Work out the finished part from the listing and answer in its coordinate system (mm). Round coordinates to 2 decimals unless told otherwise and drop trailing zeros. Order: outer loops, then holes, each group sorted by start corner. A loop starts at its lowest first (then second) coordinate and runs counter-clockwise, first axis right, second up. Notation, with made-up numbers: M -39.5,68 L -12.5,68 A10 cw -12.5,72 Z; hole C -31,11 d2. An arc over 180 degrees is marked long. Return JSON: item names as keys, results as strings.
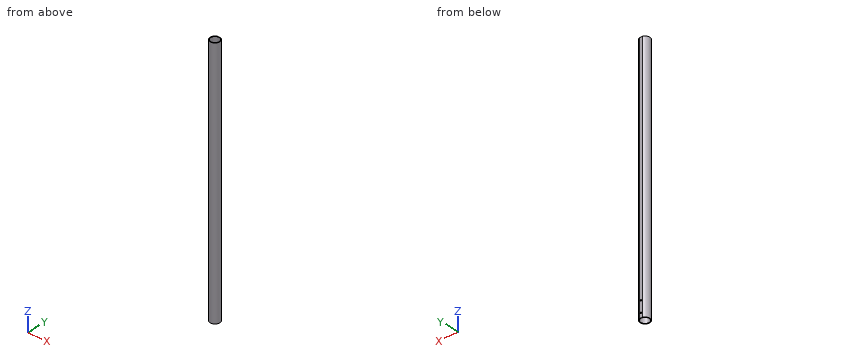
Autodesk Inventor part; units mm, degrees
ref_plane "YZ Plane" through (0, 0, 0) normal (1, 0, 0) x (0, 1, 0)
ref_plane "XZ Plane" through (0, 0, 0) normal (0, 1, 0) x (-1, 0, 0)
ref_plane "XY Plane" through (0, 0, 0) normal (0, 0, 1) x (1, 0, 0)
sketch "Sketch1" plane through (0, 0, 0) normal (0, 0, 1) x (1, 0, 0)
  circle A0 centre (0, 0) radius 11
  circle A1 centre (0, 0) radius 9.38
  dimension "d0" = 22
  dimension "d2" = 1.62
extrude "Extrusion1" add sketch "Sketch1" along normal blind 560
sketch "Sketch6" plane through (0, 0, 560) normal (0, 0, 1) x (1, 0, 0)
  circle A0 centre (0, 0) radius 9.38
  circle A1 centre (0, 0) radius 11
  line L0 (-3.2787, 10.5) -> (3.2787, 10.5)
  dimension "d18" = 10.5
extrude "Extrusion3" cut sketch "Sketch6" against normal through all contours L0 A1 picked at (-0.3693, 10.648)
sketch "Sketch8" plane through (-3.2787, 10.5, 560) normal (0, 1, 0) x (1, 0, 0)
  circle A0 centre (3.2787, 550) radius 1.7934
  point P0 (3.2787, 560)
  dimension "d47" = 10
hole "Hole4" at (0, 10.5, 10) direction (0, -1, 0) diameter 3 depth 8 tip angle 118
sketch "Sketch9" plane through (-3.2787, 10.5, 560) normal (0, 1, 0) x (1, 0, 0)
  circle A0 centre (3.2787, 550) radius 1.5
  circle A1 centre (3.2787, 525) radius 1.2403
  point P0 (3.2787, 560)
  dimension "d55" = 25
hole "Hole5" at (0, 10.5, 35) direction (0, -1, 0) diameter 3 depth 8 tip angle 118
properties part number "2f2barm" material "PVC-Piping"
Item 1: Each of these flat-tipped pins is pushed along its axis until it touches: pin 1 (2.5 mm diameter, centred on x = 0, z = 35, fed in from +Y); pin 2 (4 mm diameter, centred on y = -7, z = 440, fed in from +X); pin 3 (5 mm diameter, centred on y = 4, z = 300.5, fed in from -X). Where does it stop, or does it pass through?
Output:
{"pin 1": "stops at y = -9.3", "pin 2": "stops at x = 9.8", "pin 3": "stops at x = -10.9"}
Item 2: Consider line 1 along Z through (x, y) = (0, 9.95); line 2 along X through (y, z) = (0.25, 258); line 3 along Y through (x, z) = (0, 310.5). Determine where each line is inside the solid, lowest interval first. Write a range as [from, to].
Output:
{"line 1": "z = [0, 8.5], [11.5, 33.5], [36.5, 560]", "line 2": "x = [-11, -9.38], [9.38, 11]", "line 3": "y = [-11, -9.38], [9.38, 10.5]"}
Item 3: Find section A-A (y = 0). Determine the outline of the cut face in (x, z).
Output:
{"outline": "M -11,0 L -9.38,0 L -9.38,560 L -11,560 Z; M 9.38,0 L 11,0 L 11,560 L 9.38,560 Z"}
Item 4: Find section B-B (z = 41.5). Determine the outline of the cut face in (x, y), plus the area to 3 significant figures.
Output:
{"outline": "M -3.28,10.5 A11 ccw long 3.28,10.5 Z; hole C 0,0 d18.76", "area": "102 mm^2"}
